Can you work these out from the drawing? Everything is in mm from the part's minimum corner. A direction names the side the tool comes from. Give positions to 0.01 mm unless a question says otherwise; leave off trailing zeros. Order: outer loops, then holes, each group sorted by start corner. A loop starts at its lowest first (then second) coordinate and runs counter-clockwise, first axis right, second up. Notation, with made-up numbers: (49.5, 64) - (82.5, 64) arc R16 cw to (82.5, 77) - close; hole circle Ø5 at (-18, 23). An arc over 180 degrees is marked (long way). One line per question, with ' | ' between items.
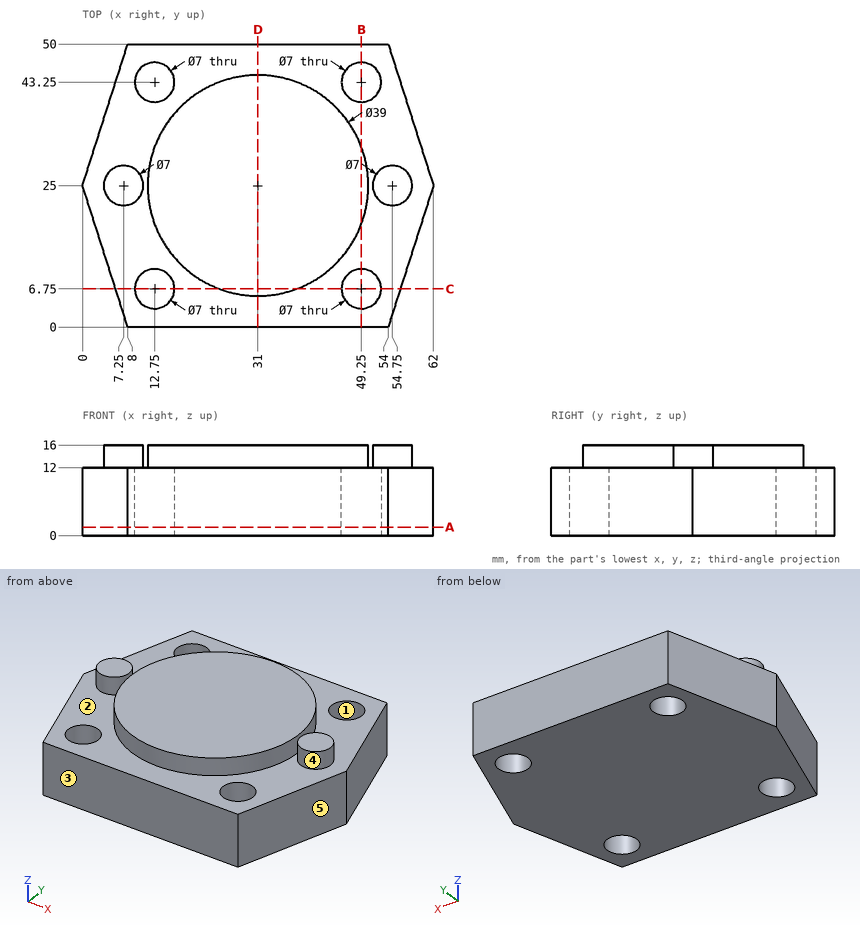
1) I want a section at D-D (x = 31). List the corners of the cut face in (y, z) for me.
Model answer:
outline: (0, 0) - (50, 0) - (50, 12) - (44.5, 12) - (44.5, 16) - (5.5, 16) - (5.5, 12) - (0, 12) - close
2) Thinking about a two-plate mould opening in X: for the marked faces 3, 4 and 5, which applies, +X half, -X half, draft (parallel to the pull), parting line (faces both ways), or undercut?
Model answer:
face 3: draft | face 4: undercut | face 5: +X half
3) On a 3-axis mill with a long thin cutter (end or side, diameter ignored), from which of +Z, -Z, +X, -X, +Y, -Y can I reach the whole of each face in a straight line? I mean the marked faces 1 and 2. Say none if no direction works.
Model answer:
face 1: +Z, -Z | face 2: +Z
4) Please list where these lines run through material, in increasing order: L1, parallel to Y at x = 49.25, z = 3.5; L2, parallel to X at y = 42.5, z = 10; L3, parallel to Y at x = 47.5, z = 3.
Model answer:
L1: y = 0 to 3.25, 10.25 to 39.75, 46.75 to 50 | L2: x = 5.6 to 9.33, 16.17 to 45.83, 52.67 to 56.4 | L3: y = 0 to 3.72, 9.78 to 40.22, 46.28 to 50
5) I'm going to push flat-ended pins straight in: P1, Ø11, axis at x = 49.25, y = 6.75, coming from the +Z side; P2, Ø6, axis at y = 42.5, z = 6, coming from the +X side. Where does each tip first touch, or does it pass through?
Model answer:
P1: stops at z = 12 | P2: stops at x = 57.36
6) I want a section at A-A (z = 1.5). List the corners of the cut face in (x, y) for me.
Model answer:
outline: (0, 25) - (8, 0) - (54, 0) - (62, 25) - (54, 50) - (8, 50) - close; hole circle Ø7 at (12.75, 6.75); hole circle Ø7 at (12.75, 43.25); hole circle Ø7 at (49.25, 6.75); hole circle Ø7 at (49.25, 43.25)
7) I want a section at C-C (y = 6.75). List the corners of the cut face in (x, z) for me.
Model answer:
outline: (5.84, 0) - (9.25, 0) - (9.25, 12) - (5.84, 12) - close; (16.25, 0) - (45.75, 0) - (45.75, 12) - (37.87, 12) - (37.87, 16) - (24.13, 16) - (24.13, 12) - (16.25, 12) - close; (52.75, 0) - (56.16, 0) - (56.16, 12) - (52.75, 12) - close
8) I want a section at B-B (x = 49.25). List the corners of the cut face in (y, z) for me.
Model answer:
outline: (0, 0) - (3.25, 0) - (3.25, 12) - (0, 12) - close; (10.25, 0) - (39.75, 0) - (39.75, 12) - (31.87, 12) - (31.87, 16) - (18.13, 16) - (18.13, 12) - (10.25, 12) - close; (46.75, 0) - (50, 0) - (50, 12) - (46.75, 12) - close
